Study the drawing (mm; zero at the part's minimum x, y, z) and answer. Round coordinates to 2 decimals unless told otherwise and drop trailing zeros. Write each loop counter-clockwise with the first axis right and the second up, starting at its lowest first coordinate (ties: lowest second). Pieces come first, ordered by that corner, then holes.
(1) Find the intervals of material crossed by probe 1 along Z at (x, y) = (9, 0.6); probe 2 along X at (y, z) = (0.75, 36.5); probe 3 along X at (y, z) = (1.05, 28), in increasing order.
(2) A cutting plane is placed at A-A, the plane z = 9. Give the vertices of the cut face in (x, y), and give its area (3 significant figures).
(3) A cutting plane is placed at C-C, the plane y = 1.1. Give the vertices of the cut face in (x, z).
(4) A cutting plane is placed at B-B, the plane z = 22.5. Give the vertices of the cut face in (x, y).
(5) A cutting plane is placed at D-D, the plane x = 9. Give the vertices of the cut face in (y, z), and give its area (3 significant figures).
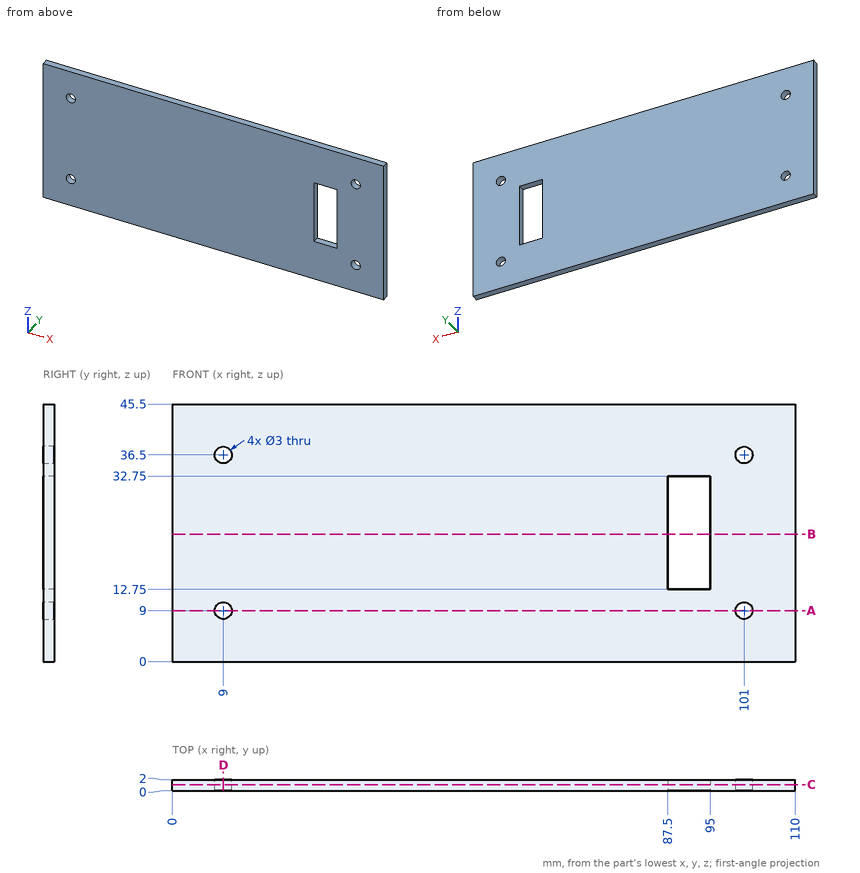
Solutions:
1. probe 1: z = 0 to 7.5, 10.5 to 35, 38 to 45.5
1. probe 2: x = 0 to 7.5, 10.5 to 99.5, 102.5 to 110
1. probe 3: x = 0 to 87.5, 95 to 110
2. outline: (0, 0) - (7.5, 0) - (7.5, 2) - (0, 2) - close; (10.5, 0) - (99.5, 0) - (99.5, 2) - (10.5, 2) - close; (102.5, 0) - (110, 0) - (110, 2) - (102.5, 2) - close
2. area: 208 mm2
3. outline: (0, 0) - (110, 0) - (110, 45.5) - (0, 45.5) - close; hole circle Ø3 at (9, 9); hole circle Ø3 at (9, 36.5); hole (87.5, 12.75) - (95, 12.75) - (95, 32.75) - (87.5, 32.75) - close; hole circle Ø3 at (101, 9); hole circle Ø3 at (101, 36.5)
4. outline: (0, 0) - (87.5, 0) - (87.5, 2) - (0, 2) - close; (95, 0) - (110, 0) - (110, 2) - (95, 2) - close
5. outline: (0, 0) - (2, 0) - (2, 7.5) - (0, 7.5) - close; (0, 10.5) - (2, 10.5) - (2, 35) - (0, 35) - close; (0, 38) - (2, 38) - (2, 45.5) - (0, 45.5) - close
5. area: 79.0 mm2
